Verification items for the finished model (mm, model axes). Round coordinates to 2 decimals unless told otherwise and drop trailing zeros. Write each loop counter-clockwise with the first axis right and the second up, starting at its lowest first coordinate (ties: lowest second). Pieces come first, ordered by that corner, then holes. Notation, with made-up numbers: M 32,16.25 L 74,16.25 A16 cw 74,44.25 Z; hole C 80.5,51 d9. An arc over 180 degrees is marked long. One line per question, with ' | ' between items.
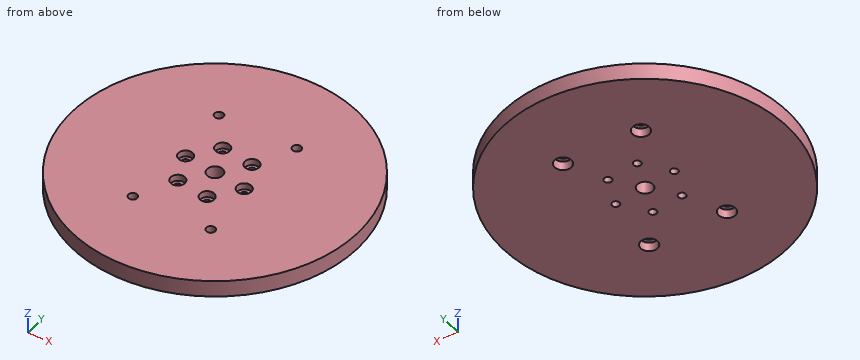
from build123d import *

# Parameters (mm, degrees)
DISCO_START                  = 420
SK_DISCO_R                   = 55
DISCO_DEPTH                  = 6.35
PASANTES_M2_5_ROTOR_J4_START = 420
SK_PASANTES_M2_5_ROTOR_J4_R  = 1.45
PASANTES_M2_5_ROTOR_J4_DEPTH = 6.35
CAJAS_M2_5_START             = 423.85
SK_CAJAS_M2_5_R              = 2.75
CAJAS_M2_5_DEPTH             = 2.5
PASO_CABLE_START             = 420
SK_PASO_CABLE_R              = 3
PASO_CABLE_DEPTH             = 6.35
SK_PASANTES_M3_PAREDES_R     = 1.7
PASANTES_M3_PAREDES_DEPTH    = 79.040518322
SK_CAJAS_M3_PAREDES_R        = 3.25
CAJAS_M3_PAREDES_DEPTH       = 3.5


with BuildPart() as part:
    # Sk_Disco → Disco (new body)
    with BuildSketch(Plane.XY.offset(DISCO_START)):
        Circle(SK_DISCO_R)
    extrude(amount=DISCO_DEPTH)

    # Sk_Pasantes_M2-5_rotor_J4 → Pasantes_M2-5_rotor_J4 (cut)
    with BuildSketch(Plane.XY.offset(PASANTES_M2_5_ROTOR_J4_START)):
        with Locations((12.390194253, -1.653204878)):
            Circle(SK_PASANTES_M2_5_ROTOR_J4_R)
        with Locations((7.626814549, 9.903620542)):
            Circle(SK_PASANTES_M2_5_ROTOR_J4_R)
        with Locations((-4.763379704, 11.55682542)):
            Circle(SK_PASANTES_M2_5_ROTOR_J4_R)
        with Locations((-12.390194253, 1.653204878)):
            Circle(SK_PASANTES_M2_5_ROTOR_J4_R)
        with Locations((-7.626814549, -9.903620542)):
            Circle(SK_PASANTES_M2_5_ROTOR_J4_R)
        with Locations((4.763379704, -11.55682542)):
            Circle(SK_PASANTES_M2_5_ROTOR_J4_R)
    extrude(amount=PASANTES_M2_5_ROTOR_J4_DEPTH, mode=Mode.SUBTRACT)

    # Sk_Cajas_M2-5 → Cajas_M2-5 (cut)
    with BuildSketch(Plane.XY.offset(CAJAS_M2_5_START)):
        with Locations((12.390194253, -1.653204878)):
            Circle(SK_CAJAS_M2_5_R)
        with Locations((7.626814549, 9.903620542)):
            Circle(SK_CAJAS_M2_5_R)
        with Locations((-4.763379704, 11.55682542)):
            Circle(SK_CAJAS_M2_5_R)
        with Locations((-12.390194253, 1.653204878)):
            Circle(SK_CAJAS_M2_5_R)
        with Locations((-7.626814549, -9.903620542)):
            Circle(SK_CAJAS_M2_5_R)
        with Locations((4.763379704, -11.55682542)):
            Circle(SK_CAJAS_M2_5_R)
    extrude(amount=CAJAS_M2_5_DEPTH, mode=Mode.SUBTRACT)

    # Sk_Paso_cable → Paso_cable (cut)
    with BuildSketch(Plane.XY.offset(PASO_CABLE_START)):
        Circle(SK_PASO_CABLE_R)
    extrude(amount=PASO_CABLE_DEPTH, mode=Mode.SUBTRACT)

    # Sk_Pasantes_M3_paredes → Pasantes_M3_paredes (cut, through all)
    with BuildSketch(Plane.XY.offset(426.35)):
        with Locations((-15, -24.675)):
            Circle(SK_PASANTES_M3_PAREDES_R)
        with Locations((15, -24.675)):
            Circle(SK_PASANTES_M3_PAREDES_R)
        with Locations((-15, 24.675)):
            Circle(SK_PASANTES_M3_PAREDES_R)
        with Locations((15, 24.675)):
            Circle(SK_PASANTES_M3_PAREDES_R)
    extrude(amount=-PASANTES_M3_PAREDES_DEPTH, mode=Mode.SUBTRACT)

    # Sk_Cajas_M3_paredes → Cajas_M3_paredes (cut)
    with BuildSketch(Plane(origin=(0, 0, 420), x_dir=(-1, 0, 0), z_dir=(0, 0, -1))):
        with Locations((15, -24.675)):
            Circle(SK_CAJAS_M3_PAREDES_R)
        with Locations((-15, -24.675)):
            Circle(SK_CAJAS_M3_PAREDES_R)
        with Locations((15, 24.675)):
            Circle(SK_CAJAS_M3_PAREDES_R)
        with Locations((-15, 24.675)):
            Circle(SK_CAJAS_M3_PAREDES_R)
    extrude(amount=-CAJAS_M3_PAREDES_DEPTH, mode=Mode.SUBTRACT)


solid = part.part
1. Section check D-D, the plane x = 43. Record the cut outline in (y, z).
Results:
outline: M -34.29,420 L 34.29,420 L 34.29,426.35 L -34.29,426.35 Z
2. Go/stop test with flat-tipped pins: P1, Ø6, axis at x = 15, y = -24.675, coming from the -Z side; P2, Ø2, axis at y = 25, z = 423.5, coming from the +X side; P3, Ø2, axis at x = 4, z = 421.5, coming from the +Y side. Record where each tip stops, or that it passes through.
Results:
P1: stops at z = 423.5 | P2: stops at x = 49.49 | P3: stops at y = 54.92
3. Section check A-A, the plane x = 0. Record the cut outline in (y, z).
Results:
outline: M -55,420 L -3,420 L -3,426.35 L -55,426.35 Z; M 3,420 L 55,420 L 55,426.35 L 3,426.35 Z
4. Section check C-C, the plane x = -20.5. Record the cut outline in (y, z), then the cut area to 3 significant figures.
Results:
outline: M -51.04,420 L 51.04,420 L 51.04,426.35 L -51.04,426.35 Z | area: 648 mm2
5. Thickness scan on line 1 (X direction, y = 25, z = 425.25); line 2 (Y direction, x = -8.5, z = 424.5); line 3 (Y direction, x = 13.5, z = 424.5) (3 decimals). Record the ranges inside material, lowest first.
Results:
line 1: x = -48.99 to -16.67, -13.33 to 13.33, 16.67 to 48.99 | line 2: y = -54.34 to -12.51, -7.3 to 54.34 | line 3: y = -53.317 to -25.475, -23.875 to -4.169, 0.863 to 23.875, 25.475 to 53.317
6. Section check B-B, the plane z = 421. Count the separate pieces of the cut face and the enclosed holes in it, then the cut area to 3 significant figures.
Results:
separate pieces: 1 | enclosed holes: 11 | area: 9,300 mm2
